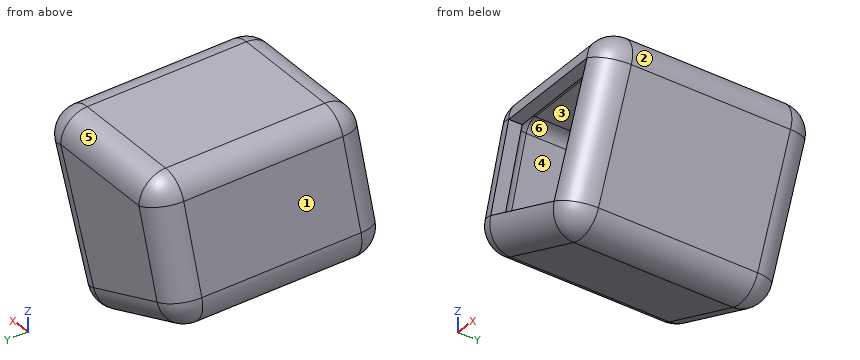
```python
from build123d import *

# Parameters (mm, degrees)
F1_DEPTH = 50.8
F2_R     = 12.7
F3_T     = -6.35


# Not quite as in the source:
# - a shell that OpenCascade refuses in one call is made with other operations: the cavity is built on its own and cut out


with BuildPart() as f1:
    # F0 (on Front) → F1 (new body, symmetric)
    with BuildSketch(Plane.XZ):
        Polygon((36.0003995515, 21.6075032949), (-44.0155640244, 21.6075032949), (-62.2989119761, -37.2344391203), (2.6374720037, -62.877625227), align=None)
    extrude(amount=F1_DEPTH, both=True)

    # F2
    f2_edges = [f1.edges().sort_by_distance(p)[0] for p in [
        (36.0004, 0, 21.607503),
        (-4.007582, 50.8, 21.607503),
        (-44.015564, 0, 21.607503),
        (-4.007582, -50.8, 21.607503),
        (19.318936, -50.8, -20.635061),
        (-53.157238, -50.8, -7.813468),
        (-29.83072, -50.8, -50.056032),
        (19.318936, 50.8, -20.635061),
        (2.637472, 0, -62.877625),
        (-53.157238, 50.8, -7.813468),
        (-29.83072, 50.8, -50.056032),
        (-62.298912, 0, -37.234439),
    ]]
    fillet(f2_edges, radius=F2_R)

    # F3: a shell. OpenCascade refuses it in one call, so the cavity is built on its own and cut out:
    # the body offset inwards by the wall thickness, plus a prism from it out through each open face.
    f3_core = offset(f1.part, amount=F3_T, mode=Mode.PRIVATE)
    f3_exits = [f3_core.faces().sort_by_distance(p)[0] for p in [
        (-15.577686, -44.45, -14.539718),
    ]]
    add(f3_core, mode=Mode.SUBTRACT)
    extrude(f3_exits, amount=-F3_T, mode=Mode.SUBTRACT)


solid = f1.part
```
Model file for the job. Use its own axes, mm. Face numbers are marked on the shaded views. A direction names the side the tool comes from. Coordinates: 2 decimals unless noted, no trailing zeros. Loops run counter-clockwise (first coordinate to the right, second up) from the corner with the lowest first, then second, coordinate; pieces in that order, holes last. Notation, with made-up numbers: (-17.5, 6) - (22.5, 6) arc R18 cw to (22.5, 12) - close; hole circle Ø10 at (7.5, 4). An arc over 180 degrees is marked (long way). Write item = value, one per line. Start each with the question number.
Item 1: 3-axis set-ups, long thin cutter, end or side, ignore diameter. For the marked faces 5 and 6: which of +Z, -Z, +X, -X, +Y, -Y reach the whole face in a straight line?
Item 2: Wall check: probe 1 along Y at (x, z) = (-25, 1); probe 2 along Z at (x, y) = (-9, 35); probe 3 along X at (y, z) = (-36, -22.5). Give the ranges that are in metal, low to high. Write a range as [from, to].
Item 3: Drop flat-ended pins along their axis: pin 1 Ø4 at (x, z) = (7.5, 5.5) entering from -Y; pin 2 Ø1.9 at (x, y) = (-17.5, -46) entering from -Z; pin 3 Ø6 at (y, z) = (1, -44) entering from +X. Give the stop position or say it passes through.
Item 4: Pull direction X, two halves, no side cores. Call the marked faces 1, 2, 3 and 4: +X half, -X half, draft (parallel to the pull), parting line (faces both ways), or undercut.
Item 5: Saw through at A-A, the plane y = -15. List the corners of the cut face in (x, z), then the cut area to 3 significant figures.
Answers:
q1.face_5 = +Z, +X, -X, +Y
q1.face_6 = none
q2.probe_1 = [44.45, 50.8]
q2.probe_2 = [-58.28, -51.45], [15.26, 21.61]
q2.probe_3 = [-57.72, -51.07], [11.76, 18.58]
q3.pin_1 = 44.45
q3.pin_2 = -52.8
q3.pin_3 = 11.28
q4.face_1 = -X half
q4.face_2 = +X half
q4.face_3 = undercut
q4.face_4 = undercut
q5.outline = (-58.8, -25.98) arc R12.7 ccw to (-51.34, -41.56) - (-9.17, -58.21) arc R12.7 ccw to (7.3, -51.07) - (29.14, 4.24) arc R12.7 ccw to (17.33, 21.61) - (-34.66, 21.61) arc R12.7 ccw to (-46.79, 12.68) - close; hole (-52.74, -27.87) arc R6.35 ccw to (-49.01, -35.66) - (-6.84, -52.31) arc R6.35 ccw to (1.4, -48.73) - (23.24, 6.58) arc R6.35 ccw to (17.33, 15.26) - (-34.66, 15.26) arc R6.35 ccw to (-40.73, 10.79) - close
q5.area = 1,630 mm2
